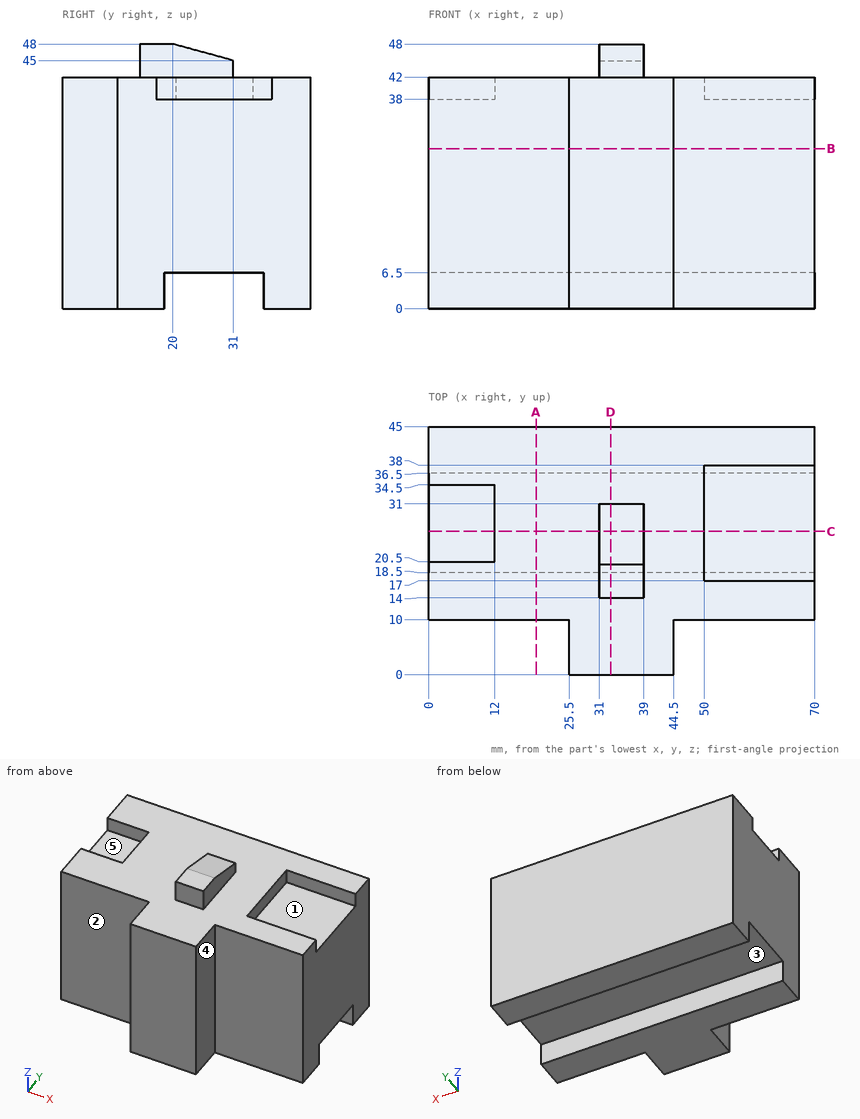
Design review of the part shown in the three views and the two pictorial views. Dimensions are in mm from the part's minimum x, y and z. A direction names the side the tool comes from. Give positions to 0.01 mm unless a question says otherwise; leave off trailing zeros. Loops run counter-clockwise (first coordinate to the right, second up) from the corner with the lowest first, then second, coordinate; pieces in that order, holes last. Notation, with made-up numbers: (-40, 35.5) - (-32, 35.5) arc R16 ccw to (-32, 42.5) - close; hole circle Ø2 at (42, -9). An arc over 180 degrees is marked (long way). Answer as a JSON object with one key per item and string values.
Q1. To check wall thickness, follow line 1 along Z through (x, y) = (35.5, 12.5); line 2 along Z through (x, y) = (61, 29.5); line 3 along X through (y, z) = (8, 40). State the ranges of each line that lie inside material, in increasing order.
Worked out:
{"line 1": "z = 0 to 42", "line 2": "z = 6.5 to 38", "line 3": "x = 25.5 to 44.5"}
Q2. For the marked faces 1, 2, 3, 4 and 5, list the 3-axis set-ups (+Z, -Z, +X, -X, +Y, -Y) from which the entire face can be reached by the end or side of a thin tool; tool diameter is ignored.
Worked out:
{"face 1": "+Z, +X", "face 2": "+Z, -Z, -X, -Y", "face 3": "-Z, +X, -X", "face 4": "+Z, -Z, +X, -Y", "face 5": "+Z, -X"}
Q3. Add section A-A on x = 19.5. State the section outline as (y, z) points.
Worked out:
{"outline": "(10, 0) - (18.5, 0) - (18.5, 6.5) - (36.5, 6.5) - (36.5, 0) - (45, 0) - (45, 42) - (10, 42) - close"}
Q4. Add section C-C on y = 26. State the section outline as (x, z) points, plus the area to 3 significant figures.
Worked out:
{"outline": "(0, 6.5) - (70, 6.5) - (70, 38) - (50, 38) - (50, 42) - (39, 42) - (39, 46.36) - (31, 46.36) - (31, 42) - (12, 42) - (12, 38) - (0, 38) - close", "area": "2,390 mm^2"}
Q5. Insertion check: pin 1 (2 mm diameter, centred on x = 3.5, z = 39.5, fed in from -Y); pin 2 (3 mm diameter, centred on y = 26.5, z = 46, fed in from +X); pin 3 (12 mm diameter, centred on x = 60, y = 31.5, fed in from +Z). Each pin has a flat end and moves straight along its axis. Give the tip position at first contact, or say it passes through.
Worked out:
{"pin 1": "stops at y = 10", "pin 2": "stops at x = 39", "pin 3": "stops at z = 38"}
Q6. Add section D-D on x = 33. State the section outline as (y, z) points, plus the area to 3 significant figures.
Worked out:
{"outline": "(0, 0) - (18.5, 0) - (18.5, 6.5) - (36.5, 6.5) - (36.5, 0) - (45, 0) - (45, 42) - (31, 42) - (31, 45) - (20, 48) - (14, 48) - (14, 42) - (0, 42) - close", "area": "1,860 mm^2"}
Q7. Add section B-B on z = 29. State the section outline as (x, y) points.
Worked out:
{"outline": "(0, 10) - (25.5, 10) - (25.5, 0) - (44.5, 0) - (44.5, 10) - (70, 10) - (70, 45) - (0, 45) - close"}
